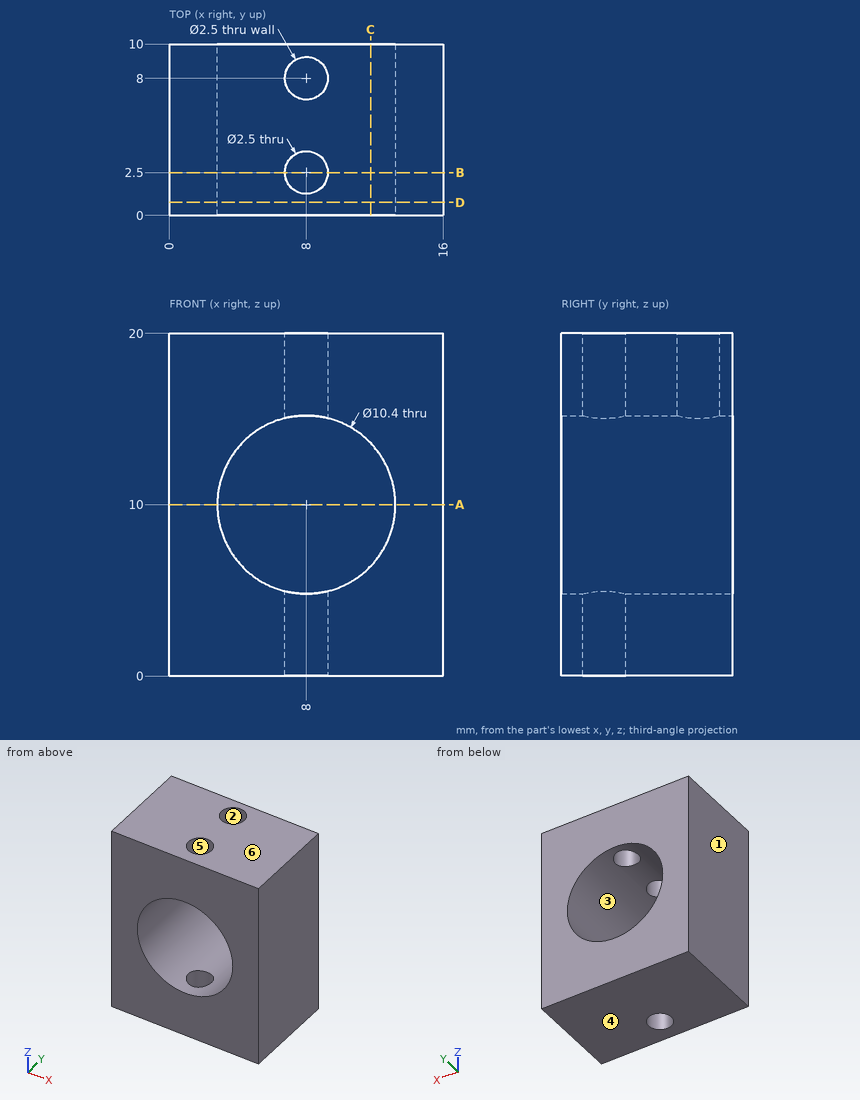
Check sheet for the drawn part. Datum: minimum x, y, z corner. Units: mm. A direction names the side the tool comes from. Round coordinates to 2 decimals unless told otherwise and drop trailing zeros. Loops run counter-clockwise (first coordinate to the right, second up) from the corner with the lowest first, then second, coordinate; pieces in that order, holes last. Notation, with made-up numbers: (35, -27.75) - (53, -27.75) arc R16 cw to (53, 0.25) - close; hole circle Ø4 at (0.25, 82.25). An arc over 180 degrees is marked (long way). Write item = value, one per line. Start each with the question number.
1. Section check B-B on y = 2.5. Enter the section's corners in (x, z).
2. Set-up check for the marked faces 1 and 2: record each of +Z, -Z, +X, -X, +Y, -Y from which the full face is reachable in a straight line by a thin tool's end or side.
3. Depth check by flat-ended pin: pin 1 (2 mm diameter, centred on x = 8, y = 8, fed in from +Z). Enter the tip coordinate at first touch or a pass-through.
4. Thickness scan on line 1 (Y direction, x = 8, z = 16.95); line 2 (Z direction, x = 8, y = 6.5); line 3 (Y direction, x = 8, z = 1.2). Record the ranges inside material, lowest first.
5. Section check C-C on x = 11.75. Enter the section's corners in (y, z).
6. Mould release check, pull along Z, two halves, no side actions. Record for the marked faces 3, 4, 5 and 6: released by +Z, released by -Z, zero draft, split by the parting line, or undercut.
7. Section check D-D on y = 0.75. Enter the section's corners in (x, z), then the cut area to 3 significant figures.
8. Section check A-A on z = 10. Enter the section's corners in (x, y).
Working result:
q1.outline = (0, 0) - (6.75, 0) - (6.75, 4.95) arc R5.2 cw to (6.75, 15.05) - (6.75, 20) - (0, 20) - close; (9.25, 0) - (16, 0) - (16, 20) - (9.25, 20) - (9.25, 15.05) arc R5.2 cw to (9.25, 4.95) - close
q2.face_1 = +Z, -Z, -X, +Y, -Y
q2.face_2 = +Z
q3.pin_1 = 4.9
q4.line_1 = 0 to 1.25, 3.75 to 6.75, 9.25 to 10
q4.line_2 = 0 to 4.8, 15.2 to 20
q4.line_3 = 0 to 1.25, 3.75 to 10
q5.outline = (0, 0) - (10, 0) - (10, 6.4) - (0, 6.4) - close; (0, 13.6) - (10, 13.6) - (10, 20) - (0, 20) - close
q6.face_3 = undercut
q6.face_4 = released by -Z
q6.face_5 = zero draft
q6.face_6 = released by +Z
q7.outline = (0, 0) - (16, 0) - (16, 20) - (0, 20) - close; hole circle Ø10.4 at (8, 10)
q7.area = 235 mm^2
q8.outline = (0, 0) - (2.8, 0) - (2.8, 10) - (0, 10) - close; (13.2, 0) - (16, 0) - (16, 10) - (13.2, 10) - close
